```python
from build123d import *

# Parameters (mm, degrees)
POCKET_DEPTH       = 118.917408
POLARPATTERN_COUNT = 36
CHAMFER_SIZE       = 0.5


with BuildPart() as part:
    # Sketch → Revolution (revolve)
    with BuildSketch(Plane.XZ):
        Polygon((0, 0), (0, 15.3), (17.5, 15.3), (17.5, 11.8), (4, 11.8), (4, 2.5), (2.5, 2.5), (2.5, 0), align=None)
    revolve(axis=Axis((0, 0, 0), (0, 0, 1)))

    # Sketch001 → Pocket (cut, through all)
    with BuildSketch(Plane.XY.offset(15.3)):
        Polygon((-0.154839, 4), (-0.6, 15.5), (0.6, 15.5), (0.154839, 4), align=None)
    pocket = extrude(amount=-POCKET_DEPTH, mode=Mode.SUBTRACT)

    # PolarPattern: Pocket ×36 about axis
    polarpattern_axis = Axis((0, 0, 15.3), (0, 0, 1))
    for i in range(1, POLARPATTERN_COUNT):
        add(pocket.rotate(polarpattern_axis, i * 360 / POLARPATTERN_COUNT), mode=Mode.SUBTRACT)

    # Chamfer
    chamfer_edges = [part.edges().sort_by_distance(p)[0] for p in [
        (-17.5, 0, 11.8),
        (-17.5, 0, 15.3),
    ]]
    chamfer(chamfer_edges, length=CHAMFER_SIZE)


solid = part.part
```
Build history of the part. All positions in model axes, mm. Give positions to 0.01 mm unless a question says otherwise; leave off trailing zeros. Loops run counter-clockwise (first coordinate to the right, second up) from the corner with the lowest first, then second, coordinate; pieces in that order, holes last.
1) Drop a flat-ended pin along its axis: P1, Ø5, axis at x = -4.5, y = 5.5, coming from the -Z side. Give the stop position or say it passes through.
Values follow:
P1: stops at z = 11.8
2) Probe line 1 along Z through (x, y) = (10, -7.5); line 2 along Z through (x, y) = (-11.5, -13); line 3 along X through (y, z) = (-2, 10.75). List the from-to ranges inside material, lowest first.
Values follow:
line 1: z = 11.8 to 15.3
line 2: z = 12.16 to 14.94
line 3: x = -3.46 to 3.46
3) Band-saw the part on B-B on x = -9. State how many separate pieces and enclosed holes the cut face has, then the cut area to 3 significant figures.
Values follow:
separate pieces: 12
enclosed holes: 0
area: 64.8 mm2
4) Two-plate mould, pull along Y, no slides. Class faces 1 (the face through (-9.11, 3.72, 13.57)), 2 (the face through (13.43, -7.74, 13.57)): released by +Y, released by -Y, zero draft, split by the parting line, or undercut.
Values follow:
face 1: undercut
face 2: undercut
5) Band-saw the part on A-A on z = 8.5. List the corners of the cut face in (x, y), then the cut area to 3 significant figures.
Values follow:
outline: circle Ø8 at (0, 0)
area: 50.3 mm2
